Part print with two shaded views. Sizes in mm from the minimum x, y, z corner. Give positions to 0.01 mm unless a question says otherwise; leave off trailing zeros. Write each loop counter-clockwise with the first axis right and the second up, starting at its lowest first coordinate (ties: lowest second). Pieces come first, ordered by that corner, then holes. Notation, with made-up numbers: (58, 78.5) -> (69, 78.5) arc R14 cw to (69, 91.5) -> close; hole circle Ø1 at (-12.5, -31.5). An arc over 180 degrees is marked (long way). Write item = value, one per line. Start each with the question number.
Q1. Saw through at D-D, the plane x = 69. List the corners of the cut face in (y, z).
Q2. Saw through at A-A, the plane x = 39.25. List the corners of the cut face in (y, z).
Q3. Saw through at C-C, the plane y = 2.95. List the corners of the cut face in (x, z).
Q4. Wall check: line 1 (Y direction, x = 54.5, z = 11); line 2 (X direction, y = 4.15, z = 37.5); line 3 (Z direction, x = 41.5, y = 3). Give the ranges that are in metal, low to high.
Q5. Saw through at B-B, the plane z = 37.5. List the corners of the cut face in (x, y), then the cut area to 3 significant figures.
Q6. Drop flat-ended pins along their axis: P1, Ø8, axis at x = 35, z = 35.5, coming from the +Y side; P2, Ø5, axis at x = 42.5, z = 31, coming from the +Y side. Give the stop position or say it passes through.
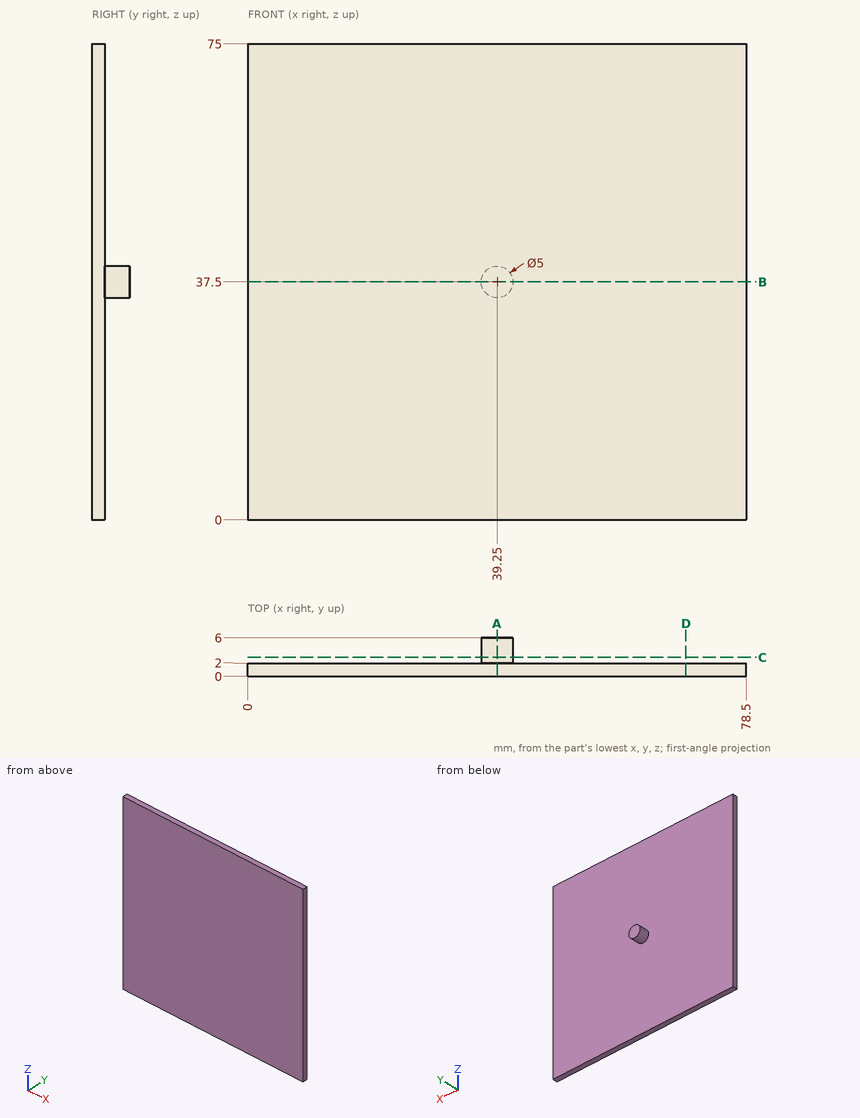
Report:
q1.outline = (0, 0) -> (2, 0) -> (2, 75) -> (0, 75) -> close
q2.outline = (0, 0) -> (2, 0) -> (2, 35) -> (6, 35) -> (6, 40) -> (2, 40) -> (2, 75) -> (0, 75) -> close
q3.outline = circle Ø5 at (39.25, 37.5)
q4.line_1 = 0 to 2
q4.line_2 = 36.75 to 41.75
q4.line_3 = 36.41 to 38.59
q5.outline = (0, 0) -> (78.5, 0) -> (78.5, 2) -> (41.75, 2) -> (41.75, 6) -> (36.75, 6) -> (36.75, 2) -> (0, 2) -> close
q5.area = 177 mm2
q6.P1 = 6
q6.P2 = 2
